from build123d import *

# Parameters (mm, degrees)
SKETCH_4_W          = 6
SKETCH_4_H          = 20
EXTRUDE_1_DEPTH     = 2
EXTRUDE_START       = -2
SKETCH_6_R          = 3.5
SKETCH_6_R_2        = 1.5
EXTRUDE_3_DEPTH     = 2
SKETCH_7_R          = 1
CUT_EXTRUDE_1_DEPTH = 12.800423721


with BuildPart() as part:
    # 草图4 → 凸台-拉伸1 (new body)
    with BuildSketch(Plane(origin=(0, 0, 0), x_dir=(1, 0, 0), z_dir=(0, 1, 0))):
        Rectangle(SKETCH_4_W, SKETCH_4_H)
    extrude(amount=EXTRUDE_1_DEPTH)

    # 草图6 → 凸台-拉伸3 (add)
    with BuildSketch(Plane.ZY.offset(3).offset(EXTRUDE_START)):
        with Locations((0, 4)):
            Circle(SKETCH_6_R)
        with Locations((0, 4)):
            Circle(SKETCH_6_R_2, mode=Mode.SUBTRACT)
    extrude(amount=-EXTRUDE_3_DEPTH)

    # 草图7 → 切除-拉伸1 (cut, through all)
    with BuildSketch(Plane(origin=(0, 2, 0), x_dir=(1, 0, 0), z_dir=(0, 1, 0))):
        with Locations(Location((0, -7.5, 0), (0, 0, 270))):
            Circle(SKETCH_7_R)
        with Locations(Location((0, 7.5, 0), (0, 0, 270))):
            Circle(SKETCH_7_R)
    extrude(amount=-CUT_EXTRUDE_1_DEPTH, mode=Mode.SUBTRACT)


solid = part.part
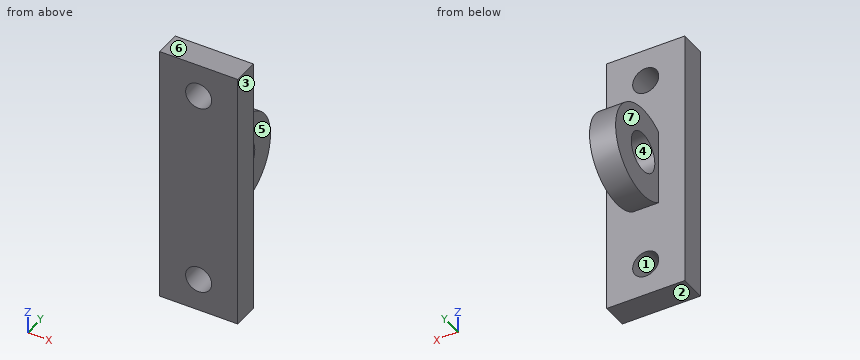
Source: CAD feature listing. Evaluate the final solid. Frame: model axes, mm. Face numbers are marked on the shaded views. A direction names the side the tool comes from. Round coordinates to 2 decimals unless told otherwise and drop trailing zeros. Order: outer loops, then holes, each group sorted by start corner. A loop starts at its lowest first (then second) coordinate and runs counter-clockwise, first axis right, second up. Notation, with made-up numbers: (-9, 73.25) - (44, 73.25) arc R11 ccw to (44, 77.25) - close; hole circle Ø3 at (-6.5, -5). An arc over 180 degrees is marked (long way). Use a Markdown table: item, result. Add a question column.
1. Section query B-B (y = 4). Return the cut outline in (x, z), then the cut area to 3 significant figures.
2. Line query: probe 1 along X at (y, z) = (1.3, -7.5); probe 2 along Y at (x, z) = (-1.05, 7.75); probe 3 along X at (y, z) = (3.25, -2.25). Output: solid intervals per line, ascending.
3. Section query A-A (z = 0). Return the cut outline in (x, y).
4. Section query D-D (z = -7.5). Return the cut outline in (x, y), then the cut area to 3 significant figures.
5. First-contact query: pin 1 (1 mm diameter, centred on x = -1, y = 5.5, fed in from +Z); pin 2 (3 mm diameter, centred on y = 4.5, z = -1, fed in from +X); pin 3 (3 mm diameter, centred on x = 2, z = 1.5, fed in from +Y). Flat tips, straight axial feed; report the tip coordinate or a pass-through.
6. Set-up query: the marked faces 5, 6 and 7. Return all of +Z, -Z, +X, -X, +Y, -Y with unobstructed straight access to the full face (end or side cutting, diameter ignored); none if empty.
7. Mould query, pull axis Z, two halves, no side actions, for the marked faces 1, 2, 3 and 4. Classes: +Z half, -Z half, draft (parallel to the pull), parting line (faces both ways), or undercut.
8. Section query C-C (x = 0). Return the cut outline in (y, z), then the cut area to 3 significant figures.
Derived:
| question | item | result |
|---|---|---|
| 1 | outline | (-1, -3.5) - (1, -3.5) - (1, -1.5) - (-1, -1.5) - close; (-1, 1.5) - (1, 1.5) - (1, 3.5) - (-1, 3.5) - close |
| 1 | area | 8.00 mm2 |
| 2 | probe 1 | -3 to -1, 1 to 3 |
| 2 | probe 2 | 0 to 2 |
| 2 | probe 3 | -1 to 1 |
| 3 | outline | (-3, 0) - (3, 0) - (3, 2) - (1, 2) - (1, 2.5) - (-1, 2.5) - (-1, 2) - (-3, 2) - close; (-1, 5.5) - (1, 5.5) - (1, 7.5) - (-1, 7.5) - close |
| 4 | outline | (-3, 0) - (-1, 0) - (-1, 2) - (-3, 2) - close; (1, 0) - (3, 0) - (3, 2) - (1, 2) - close |
| 4 | area | 8.00 mm2 |
| 5 | pin 1 | z = 3.35 |
| 5 | pin 2 | x = 1 |
| 5 | pin 3 | y = 7.48 |
| 6 | face 5 | +Z, -Z, +X, +Y |
| 6 | face 6 | +Z, +X, -X, +Y, -Y |
| 6 | face 7 | +Z, -Z, -X, +Y |
| 7 | face 1 | undercut |
| 7 | face 2 | -Z half |
| 7 | face 3 | draft |
| 7 | face 4 | undercut |
| 8 | outline | (0, -10) - (2, -10) - (2, -8.5) - (0, -8.5) - close; (0, -6.5) - (2, -6.5) - (2, -2.87) arc R3.5 ccw (long way) to (2, 2.87) - (2, 6.5) - (0, 6.5) - close; (0, 8.5) - (2, 8.5) - (2, 10) - (0, 10) - close; hole circle Ø3 at (4, 0) |
| 8 | area | 57.4 mm2 |
